```python
from build123d import *

# Parameters (mm, degrees)
BOSS_EXTRUDE1_DEPTH = 6.35
SKETCH1_R           = 7.112
CUT_EXTRUDE1_DEPTH  = 6.35
SKETCH2_W           = 10.0254
SKETCH2_H           = 4.477133961
CUT_EXTRUDE2_DEPTH  = 204.051450213
LPATTERN1_COUNT     = 9
LPATTERN1_PITCH     = 20
SKETCH5_R           = 0.79375
CUT_EXTRUDE4_DEPTH  = 3.175
LPATTERN2_COUNT     = 3
LPATTERN2_PITCH     = 2.032


# Read off the part's stored shape, not the designer's step: Boss-Extrude1
with BuildPart() as part:
    # Boss-Extrude1 outline → Boss-Extrude1 (new body)
    with BuildSketch(Plane.XY):
        with BuildLine():
            Line((190, -4.490128061), (190, -1.122532015))
            ThreePointArc((190, -1.122532015), (190, 0), (191.122532015, 0))
            Line((191.122532015, 0), (200, 0))
            Line((200, 0), (200, 30))
            Line((200, 30), (191.122532015, 30))
            ThreePointArc((191.122532015, 30), (190, 30), (190, 31.122532015))
            Line((190, 31.122532015), (190, 34.490128061))
            Line((190, 34.490128061), (180, 34.490128061))
            Line((180, 34.490128061), (180, 31.122532015))
            ThreePointArc((180, 31.122532015), (180, 30), (178.877467985, 30))
            Line((178.877467985, 30), (171.122532015, 30))
            ThreePointArc((171.122532015, 30), (170, 30), (170, 31.122532015))
            Line((170, 31.122532015), (170, 34.490128061))
            Line((170, 34.490128061), (160, 34.490128061))
            Line((160, 34.490128061), (160, 31.122532015))
            ThreePointArc((160, 31.122532015), (160, 30), (158.877467985, 30))
            Line((158.877467985, 30), (151.122532015, 30))
            ThreePointArc((151.122532015, 30), (150, 30), (150, 31.122532015))
            Line((150, 31.122532015), (150, 34.490128061))
            Line((150, 34.490128061), (140, 34.490128061))
            Line((140, 34.490128061), (140, 31.122532015))
            ThreePointArc((140, 31.122532015), (140, 30), (138.877467985, 30))
            Line((138.877467985, 30), (131.122532015, 30))
            ThreePointArc((131.122532015, 30), (130, 30), (130, 31.122532015))
            Line((130, 31.122532015), (130, 34.490128061))
            Line((130, 34.490128061), (120, 34.490128061))
            Line((120, 34.490128061), (120, 31.122532015))
            ThreePointArc((120, 31.122532015), (120, 30), (118.877467985, 30))
            Line((118.877467985, 30), (111.122532015, 30))
            ThreePointArc((111.122532015, 30), (110, 30), (110, 31.122532015))
            Line((110, 31.122532015), (110, 34.490128061))
            Line((110, 34.490128061), (100, 34.490128061))
            Line((100, 34.490128061), (100, 31.122532015))
            ThreePointArc((100, 31.122532015), (100, 30), (98.877467985, 30))
            Line((98.877467985, 30), (91.122532015, 30))
            ThreePointArc((91.122532015, 30), (90, 30), (90, 31.122532015))
            Line((90, 31.122532015), (90, 34.490128061))
            Line((90, 34.490128061), (80, 34.490128061))
            Line((80, 34.490128061), (80, 31.122532015))
            ThreePointArc((80, 31.122532015), (80, 30), (78.877467985, 30))
            Line((78.877467985, 30), (71.122532015, 30))
            ThreePointArc((71.122532015, 30), (70, 30), (70, 31.122532015))
            Line((70, 31.122532015), (70, 34.490128061))
            Line((70, 34.490128061), (60, 34.490128061))
            Line((60, 34.490128061), (60, 31.122532015))
            ThreePointArc((60, 31.122532015), (60, 30), (58.877467985, 30))
            Line((58.877467985, 30), (51.122532015, 30))
            ThreePointArc((51.122532015, 30), (50, 30), (50, 31.122532015))
            Line((50, 31.122532015), (50, 34.490128061))
            Line((50, 34.490128061), (40, 34.490128061))
            Line((40, 34.490128061), (40, 31.122532015))
            ThreePointArc((40, 31.122532015), (40, 30), (38.877467985, 30))
            Line((38.877467985, 30), (31.122532015, 30))
            ThreePointArc((31.122532015, 30), (30, 30), (30, 31.122532015))
            Line((30, 31.122532015), (30, 34.490128061))
            Line((30, 34.490128061), (20, 34.490128061))
            Line((20, 34.490128061), (20, 31.122532015))
            ThreePointArc((20, 31.122532015), (20, 30), (18.877467985, 30))
            Line((18.877467985, 30), (0, 30))
            Line((0, 30), (0, 0))
            Line((0, 0), (18.877467985, 0))
            ThreePointArc((18.877467985, 0), (20, 0), (20, -1.122532015))
            Line((20, -1.122532015), (20, -4.490128061))
            Line((20, -4.490128061), (30, -4.490128061))
            Line((30, -4.490128061), (30, -1.122532015))
            ThreePointArc((30, -1.122532015), (30, 0), (31.122532015, 0))
            Line((31.122532015, 0), (38.877467985, 0))
            ThreePointArc((38.877467985, 0), (40, 0), (40, -1.122532015))
            Line((40, -1.122532015), (40, -4.490128061))
            Line((40, -4.490128061), (50, -4.490128061))
            Line((50, -4.490128061), (50, -1.122532015))
            ThreePointArc((50, -1.122532015), (50, 0), (51.122532015, 0))
            Line((51.122532015, 0), (58.877467985, 0))
            ThreePointArc((58.877467985, 0), (60, 0), (60, -1.122532015))
            Line((60, -1.122532015), (60, -4.490128061))
            Line((60, -4.490128061), (70, -4.490128061))
            Line((70, -4.490128061), (70, -1.122532015))
            ThreePointArc((70, -1.122532015), (70, 0), (71.122532015, 0))
            Line((71.122532015, 0), (78.877467985, 0))
            ThreePointArc((78.877467985, 0), (80, 0), (80, -1.122532015))
            Line((80, -1.122532015), (80, -4.490128061))
            Line((80, -4.490128061), (90, -4.490128061))
            Line((90, -4.490128061), (90, -1.122532015))
            ThreePointArc((90, -1.122532015), (90, 0), (91.122532015, 0))
            Line((91.122532015, 0), (98.877467985, 0))
            ThreePointArc((98.877467985, 0), (100, 0), (100, -1.122532015))
            Line((100, -1.122532015), (100, -4.490128061))
            Line((100, -4.490128061), (110, -4.490128061))
            Line((110, -4.490128061), (110, -1.122532015))
            ThreePointArc((110, -1.122532015), (110, 0), (111.122532015, 0))
            Line((111.122532015, 0), (118.877467985, 0))
            ThreePointArc((118.877467985, 0), (120, 0), (120, -1.122532015))
            Line((120, -1.122532015), (120, -4.490128061))
            Line((120, -4.490128061), (130, -4.490128061))
            Line((130, -4.490128061), (130, -1.122532015))
            ThreePointArc((130, -1.122532015), (130, 0), (131.122532015, 0))
            Line((131.122532015, 0), (138.877467985, 0))
            ThreePointArc((138.877467985, 0), (140, 0), (140, -1.122532015))
            Line((140, -1.122532015), (140, -4.490128061))
            Line((140, -4.490128061), (150, -4.490128061))
            Line((150, -4.490128061), (150, -1.122532015))
            ThreePointArc((150, -1.122532015), (150, 0), (151.122532015, 0))
            Line((151.122532015, 0), (158.877467985, 0))
            ThreePointArc((158.877467985, 0), (160, 0), (160, -1.122532015))
            Line((160, -1.122532015), (160, -4.490128061))
            Line((160, -4.490128061), (170, -4.490128061))
            Line((170, -4.490128061), (170, -1.122532015))
            ThreePointArc((170, -1.122532015), (170, 0), (171.122532015, 0))
            Line((171.122532015, 0), (178.877467985, 0))
            ThreePointArc((178.877467985, 0), (180, 0), (180, -1.122532015))
            Line((180, -1.122532015), (180, -4.490128061))
            Line((180, -4.490128061), (190, -4.490128061))
        make_face()
    extrude(amount=BOSS_EXTRUDE1_DEPTH)

    # Sketch1 → Cut-Extrude1 (cut)
    with BuildSketch(Plane.XY.offset(6.35)):
        with Locations((100, 15)):
            Circle(SKETCH1_R)
    extrude(amount=-CUT_EXTRUDE1_DEPTH, mode=Mode.SUBTRACT)

    # Sketch2 → Cut-Extrude2 (cut, through all)
    with BuildSketch(Plane(origin=(0, 0, 0), x_dir=(-1, 0, 0), z_dir=(0, 0, -1))):
        with Locations((-35, 32.25156108)):
            Rectangle(SKETCH2_W, SKETCH2_H)
        with Locations((-35, -2.251561081)):
            Rectangle(SKETCH2_W, SKETCH2_H)
    cut_extrude2 = extrude(amount=-CUT_EXTRUDE2_DEPTH, mode=Mode.SUBTRACT)

    # LPattern1: Cut-Extrude2 ×9
    with Locations(*[(i * LPATTERN1_PITCH, 0, 0) for i in range(1, LPATTERN1_COUNT)]):
        add(cut_extrude2, mode=Mode.SUBTRACT)

    # Sketch5 → Cut-Extrude4 (cut)
    with BuildSketch(Plane(origin=(0, 0, 0), x_dir=(-1, 0, 0), z_dir=(0, 0, -1))):
        with Locations((-2.032, 2.032)):
            Circle(SKETCH5_R)
    cut_extrude4 = extrude(amount=-CUT_EXTRUDE4_DEPTH, mode=Mode.SUBTRACT)

    # LPattern2: Cut-Extrude4 ×3
    with Locations(*[(0, i * LPATTERN2_PITCH, 0) for i in range(1, LPATTERN2_COUNT)]):
        add(cut_extrude4, mode=Mode.SUBTRACT)


solid = part.part
```
Input: part model. Units: mm. Frame: model coordinates. A direction names the side the tool comes from. Give positions to 0.01 mm unless a question says otherwise; leave off trailing zeros. Write each loop counter-clockwise with the first axis right and the second up, starting at its lowest first coordinate (ties: lowest second). Pieces come first, ordered by that corner, then holes. Notation, with made-up numbers: (87, 75.25) - (129, 75.25) arc R27 cw to (129, 110.25) - close; hole circle Ø11 at (-13.75, -33.75). An arc over 180 degrees is marked (long way). Write item = value, one per line. Start each with the question number.
1. Access query for faces 5 (the flat face through (85, 34.49, 3)), 6 (the flat face through (49.987, 33, 3)), 7 (the flat face through (175, 0, 3)), 8 (the flat face through (196, 30, 3)). Directions: +Z, -Z, +X, -X, +Y, -Y. A direction counts if a zero-diameter tool reaches every point of the face in a straight line with its end or side. Return the directions, or none.
2. First-contact query: pin 1 Ø3 at (y, z) = (22.5, 2.5) entering from -X; pin 2 Ø1 at (y, z) = (-3, 4.5) entering from -X; pin 3 Ø1 at (y, z) = (32.5, 3) entering from +X; pin 4 Ø0.5 at (x, y) = (2, 6) entering from -Z (3 decimals). Flat tips, straight axial feed; report the tip coordinate or a pass-through.
3. Section query A-A, the plane y = 15. Output: boundary loops of the cut face in (x, z).
4. Section query B-B, the plane x = 102.5. Output: boundary loops of the cut face in (y, z).
5. Ray query, L1, parallel to Y at x = 57.5, z = 3.5; L2, parallel to X at y = 13, z = 2 (3 decimals); L3, parallel to X at y = 21.5, z = 2.5. Return the intervals inside material, ascending.
6. Mould query, pull axis X, two halves, no side actions, for faces 1 (the flat face through (185, -4.49, 3)), 2 (the flat face through (175, 30, 3)), 3 (the flat face through (69.987, -3, 3)), 4 (the flat face through (189.987, -3, 3)). Classes: released by +X, released by -X, zero draft, split by the parting line, or undercut.
Check sheet entries:
q1.face_5 = +Z, -Z, +X, -X, +Y
q1.face_6 = +Z, -Z, +Y
q1.face_7 = +Z, -Z, -Y
q1.face_8 = +Z, -Z, +X, +Y
q2.pin_1 = 0
q2.pin_2 = 20
q2.pin_3 = 189.99
q2.pin_4 = 3.175
q3.outline = (0, 0) - (92.89, 0) - (92.89, 6.35) - (0, 6.35) - close; (107.11, 0) - (200, 0) - (200, 6.35) - (107.11, 6.35) - close
q4.outline = (-4.49, 0) - (8.34, 0) - (8.34, 6.35) - (-4.49, 6.35) - close; (21.66, 0) - (34.49, 0) - (34.49, 6.35) - (21.66, 6.35) - close
q5.L1 = 0 to 30
q5.L2 = 0 to 93.175, 106.825 to 200
q5.L3 = 0 to 97.11, 102.89 to 200
q6.face_1 = zero draft
q6.face_2 = undercut
q6.face_3 = undercut
q6.face_4 = released by +X
